from build123d import *

# Parameters (mm, degrees)
SKETCH1_R          = 19.05
BASE_EXTRUDE_DEPTH = 3.175


with BuildPart() as part:
    # Sketch1 → Base-Extrude (new body)
    with BuildSketch(Plane.XY):
        with BuildLine():
            Line((-752.475, -79.774296229), (-695.3504, -346.781975691))
            ThreePointArc((-695.3504, -346.781975691), (0.389674853, -273.050022898), (696.1124, -346.945505398))
            Line((696.1124, -346.945505398), (752.475, -79.774296229))
            ThreePointArc((752.475, -79.774296229), (0, 0), (-752.475, -79.774296229))
        make_face()
        with Locations((-446.3034, -108.204)):
            Circle(SKETCH1_R, mode=Mode.SUBTRACT)
        with Locations((-571.9318, -126.7714)):
            Circle(SKETCH1_R, mode=Mode.SUBTRACT)
        with BuildLine():
            Line((-527.768777415, -117.465403312), (-531.604993281, -179.217083351))
            add(Edge.make_bspline(
                [(-531.604993281, -179.217083351), (-537.072397888, -267.226056703), (-468.944973872, -245.915384382), (-400.817549855, -224.604712061), (-455.462578204, -155.39927311)],
                knots=[1.113887128, 1.113887128, 1.113887128, 3.141592654, 3.141592654, 5.169298179, 5.169298179, 5.169298179], degree=2, weights=[1, 0.52859414, 1, 0.52859414, 1]))
            Line((-455.462578204, -155.39927311), (-493.80437652, -106.841132272))
            ThreePointArc((-493.80437652, -106.841132272), (-514.442639374, -100.465315857), (-527.768777415, -117.465403312))
        make_face(mode=Mode.SUBTRACT)
    extrude(amount=-BASE_EXTRUDE_DEPTH)


solid = part.part
The listing builds one solid part. Answer for the finished solid, in the listing's coordinates (mm). Round coordinates to 2 decimals unless told otherwise and drop trailing zeros. Loops run counter-clockwise (first coordinate to the right, second up) from the corner with the lowest first, then second, coordinate; pieces in that order, holes last. Notation, with made-up numbers: M 78.5,15 L 114.5,15 A31 ccw 114.5,41 Z; hole C 63.25,-20.75 d11. An arc over 180 degrees is marked long. Write each question's results on one line, items separated by ' | '. Start each with the question number.
1) Straight lines are drawn through the part: probe 1 along X at (y, z) = (-182, -1.4); probe 2 along X at (y, z) = (-152.5, -1.4); probe 3 along Y at (x, z) = (15.5, -0.65). For each, find the intervals that lie inside material, in ascending order.
2) Find section A-A on y = -295.5. Write down the section's boundary in (x, z) (3 decimals), plus the area to 3 significant figures.
3) Find section B-B on z = -0.6. Count the separate pieces of the cut face and the enclosed holes in it, plus the area to 3 significant figures.
4) Find section C-C on x = -171.5. Write down the section's boundary in (y, z) (3 decimals).
5) Determine the mould class of faces 1 (the cylindrical face through (10.613, -0.016, -1.565)), 2 (the flat face through (-474.365, -131.46, -1.565)), 3 (the flat face through (-11, -171, -3.175)) for opening direction Y: pulls with the +Y half, pulls with the -Y half, needs draft (parallel to the pull), parting line crosses it, or undercut.
Final values:
1) probe 1: -730.6 to -531.72, -442.48 to 730.91 | probe 2: -736.92 to -529.95, -457.75 to 737.13 | probe 3: -273.09 to -0.03
2) outline: M -706.322,-3.175 L -385.19,-3.175 L -385.19,0 L -706.322,0 Z; M 385.19,-3.175 L 706.965,-3.175 L 706.965,0 L 385.19,0 Z | area: 2,040 mm²
3) separate pieces: 1 | enclosed holes: 3 | area: 386,000 mm²
4) outline: M -277.488,-3.175 L -4.1,-3.175 L -4.1,0 L -277.488,0 Z
5) face 1: pulls with the +Y half | face 2: undercut | face 3: needs draft
